```python
from build123d import *

# Parameters (mm, degrees)
F0_W     = 17
F0_H     = 17
F1_DEPTH = 11.5
F2_R     = 3.75
F3_DEPTH = 9
F4_R     = 3
F5_DEPTH = 10
F6_W     = 17
F6_H     = 4
F7_DEPTH = 4.2
F8_R     = 8.49999


# Not quite as in the source:
# - a fillet or chamfer is up to 0.001 mm smaller than in the source, because OpenCascade refuses the exact size


with BuildPart() as f1:
    # F0 (on Front) → F1 (new body)
    with BuildSketch(Plane.XZ):
        Rectangle(F0_W, F0_H)
    extrude(amount=F1_DEPTH)

    # F2 (on face) → F3 (join)
    with BuildSketch(Plane.XZ.offset(11.5)):
        Circle(F2_R)
    extrude(amount=F3_DEPTH)

    # F4 (on face) → F5 (join)
    with BuildSketch(Plane.XZ.offset(20.5)):
        Circle(F4_R)
    extrude(amount=F5_DEPTH)

    # F6 (on face) → F7 (join)
    with BuildSketch(Plane(origin=(0, 0, -8.5), x_dir=(1, 0, 0), z_dir=(0, 0, -1))):
        with Locations((0, 2)):
            Rectangle(F6_W, F6_H)
        with Locations((0, 9.5)):
            Rectangle(F6_W, F6_H)
    extrude(amount=F7_DEPTH)

    # F8 (radius 8.5 in the source; OpenCascade refuses exactly that, so slightly less here)
    f8_edges = [f1.edges().sort_by_distance(p)[0] for p in [
        (8.5, -5.75, 8.5),
        (-8.5, -5.75, 8.5),
    ]]
    fillet(f8_edges, radius=F8_R)


solid = f1.part
```
Input: part model. Units: mm. Frame: model coordinates. A direction names the side the tool comes from. Coordinates: 2 decimals unless noted, no trailing zeros. Order: outer loops, then holes, each group sorted by start corner. A loop starts at its lowest first (then second) coordinate and runs counter-clockwise, first axis right, second up. Notation, with made-up numbers: (47, -33) - (62, -33) arc R11 ccw to (62, -22) - close; hole circle Ø9 at (75, 75.5). An arc over 180 degrees is marked (long way). Put each result on its own line as item: value.
1. Line query: line 1 along Y through (x, z) = (4.25, -10); line 2 along Y through (x, z) = (-3, -4.25); line 3 along Y through (x, z) = (-3.25, 1.25). Output: solid intervals per line, ascending.
Report:
line 1: y = -11.5 to -7.5, -4 to 0
line 2: y = -11.5 to 0
line 3: y = -20.5 to 0
2. Reachability of faces 5 (the face through (0, -10, -12.7)), 6 (the face through (0, -6, -8.5)), 7 (the face through (1, -20.5, 3)) from +Z, -Z, +X, -X, +Y, -Y: full face, straight path, thin tool, end or side. Return the list, or none.
Report:
face 5: -Z, +X, -X, +Y, -Y
face 6: -Z, +X, -X
face 7: -Y
3. Draft query along Y for faces 1 (the face through (0, -2, -12.7)), 2 (the face through (0, -30.5, 0)), 3 (the face through (0, -4, -11)), 4 (the face through (0, 0, -2)). Return one class per face: pulls with the +Y half, pulls with the -Y half, needs draft (parallel to the pull), parting line crosses it, or undercut.
Report:
face 1: needs draft
face 2: pulls with the -Y half
face 3: undercut
face 4: pulls with the +Y half
4. Cut plane C-C on z = -6. Return the cut outline in (x, y).
Report:
outline: (-8.5, -11.5) - (8.5, -11.5) - (8.5, 0) - (-8.5, 0) - close
5. Contact query for flat-ended pins moving along their axis: pin 1 Ø1 at (x, y) = (1.5, -19.5) entering from -Z; pin 2 Ø1.5 at (x, y) = (1, -24.5) entering from +Z; pin 3 Ø2 at (x, z) = (6.5, -6.5) entering from -Y. Output: stop coordinate, or through.
Report:
pin 1: stops at z = -3.61
pin 2: stops at z = 2.99
pin 3: stops at y = -11.5
6. Cut plane A-A on x = 5.75. Return the cut outline in (y, z), then the cut area to 3 significant figures.
Report:
outline: (-11.5, -12.7) - (-7.5, -12.7) - (-7.5, -8.5) - (-4, -8.5) - (-4, -12.7) - (0, -12.7) - (0, 6.26) - (-11.5, 6.26) - close
area: 203 mm2
